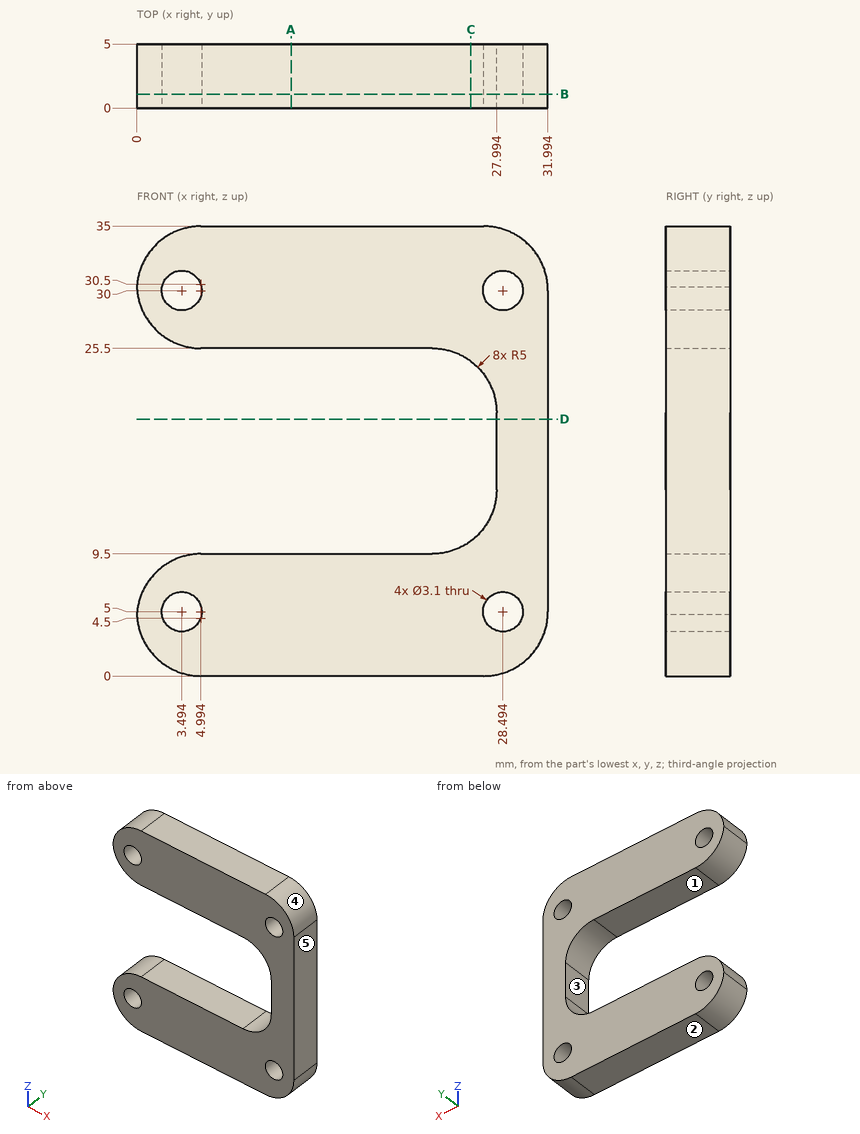
Geometry check sheet. Reference: drawing and pictorial views, mm from the part's lowest x, y, z. A direction names the side the tool comes from. Coordinates: 2 decimals unless noted, no trailing zeros. Order: outer loops, then holes, each group sorted by start corner. A loop starts at its lowest first (then second) coordinate and runs counter-clockwise, first axis right, second up. Notation, with made-up numbers: (13, 29) - (49, 29) arc R26 cw to (49, 44) - close; hole circle Ø8 at (31, 23.25). An arc over 180 degrees is marked (long way). Answer in a Markdown table with one row per item. Add a question column.
1) Cross-section at B-B, the plane y = 1.1. Record the cut outline in (x, z), then the cut area to 3 significant figures.
2) Gauge pin test, flat ends, axial feed: P1, Ø1.5, axis at y = 1.5, z = 31.5, coming from the +X side; P2, Ø2.5, axis at x = 28.49, z = 5, coming from the +Y side; P3, Ø1.5, axis at y = 4, z = 17, coming from the -X side. Record the tip position at first contact, or that the pin passes through.
3) Release check for a two-part mould opening along Z. For the marked faces 3, 4 and 5 record: +Z half, -Z half, draft (parallel to the pull), parting line (faces both ways), or undercut.
4) Material ranges on line 1 along X through (y, z) = (3.8, 5); line 2 along X through (y, z) = (1.7, 30.5); line 3 along Z through (x, y) = (10, 2.25), recorded low to high. Write a range as [from, to].
5) Set-up check for the marked faces 1 and 2: record each of +Z, -Z, +X, -X, +Y, -Y from which the full face is reachable in a straight line by a thin tool's end or side.
6) Cross-section at A-A, the plane x = 12. Record the cut outline in (y, z), then the cut area to 3 significant figures.
7) Cross-section at C-C, the plane x = 26. Record the cut outline in (y, z) (1 decimal), then the cut area to 3 significant figures.
8) Cross-section at D-D, the plane z = 20. Record the cut outline in (x, y), then the cut area to 3 significant figures.
Check result:
| question | item | result |
|---|---|---|
| 1 | outline | (0, 4.75) arc R5 ccw to (4.99, 0) - (26.99, 0) arc R5 ccw to (31.99, 5) - (31.99, 30) arc R5 ccw to (26.99, 35) - (4.99, 35) arc R5 ccw to (0, 30.25) arc R5 ccw to (4.99, 25.5) - (22.99, 25.5) arc R5 cw to (27.99, 20.5) - (27.99, 14.5) arc R5 cw to (22.99, 9.5) - (4.99, 9.5) arc R5 ccw to start; hole circle Ø3.1 at (3.49, 5); hole circle Ø3.1 at (3.49, 30); hole circle Ø3.1 at (28.49, 5); hole circle Ø3.1 at (28.49, 30) |
| 1 | area | 620 mm² |
| 2 | P1 | stops at x = 31.94 |
| 2 | P2 | passes through |
| 2 | P3 | stops at x = 27.99 |
| 3 | face 3 | undercut |
| 3 | face 4 | +Z half |
| 3 | face 5 | draft |
| 4 | line 1 | x = [0.02, 1.94], [5.04, 26.94], [30.04, 31.99] |
| 4 | line 2 | x = [0.02, 2.03], [4.96, 27.03], [29.96, 31.97] |
| 4 | line 3 | z = [0, 9.5], [25.5, 35] |
| 5 | face 1 | -X, +Y, -Y |
| 5 | face 2 | -Z, +X, -X, +Y, -Y |
| 6 | outline | (0, 0) - (5, 0) - (5, 9.5) - (0, 9.5) - close; (0, 25.5) - (5, 25.5) - (5, 35) - (0, 35) - close |
| 6 | area | 95.0 mm² |
| 7 | outline | (0, 0) - (5, 0) - (5, 10.5) - (0, 10.5) - close; (0, 24.5) - (5, 24.5) - (5, 35) - (0, 35) - close |
| 7 | area | 105 mm² |
| 8 | outline | (27.99, 0) - (31.99, 0) - (31.99, 5) - (27.99, 5) - close |
| 8 | area | 20.0 mm² |
